```python
from build123d import *

# Parameters (mm, degrees)
F0_W     = 15
F0_H     = 25
F0_R     = 2.25
F1_DEPTH = 2.5
F2_W     = 15
F2_H     = 30
F2_R     = 2.25
F3_DEPTH = 5
F4_W     = 15
F4_H     = 30
F4_R     = 2.5
F5_DEPTH = 9


with BuildPart() as f1:
    # F0 (on Top) → F1 (new body)
    with BuildSketch(Plane.XY):
        with Locations((7.5, -12.5)):
            Rectangle(F0_W, F0_H)
        with Locations((7.5, -7.405)):
            Circle(F0_R, mode=Mode.SUBTRACT)
    extrude(amount=F1_DEPTH)

    # F2 (on face) → F3 (join)
    with BuildSketch(Plane.XY.offset(2.5)):
        with Locations((7.5, -15)):
            Rectangle(F2_W, F2_H)
        with Locations((7.5, -7.405)):
            Circle(F2_R, mode=Mode.SUBTRACT)
    extrude(amount=F3_DEPTH)

    # F4 (on face) → F5 (join)
    with BuildSketch(Plane(origin=(0, 0, 0), x_dir=(1, 0, 0), z_dir=(0, 0, -1))):
        with Locations((7.5, 15)):
            Rectangle(F4_W, F4_H)
        with Locations((7.5, 7.405)):
            Circle(F4_R, mode=Mode.SUBTRACT)
    extrude(amount=F5_DEPTH)


solid = f1.part
```
Design review of the part built by this model. Coordinates are the model's own, in mm. A direction names the side the tool comes from. Round coordinates to 2 decimals unless told otherwise and drop trailing zeros. Order: outer loops, then holes, each group sorted by start corner. A loop starts at its lowest first (then second) coordinate and runs counter-clockwise, first axis right, second up. Notation, with made-up numbers: (26, 28) - (77, 28) arc R10 cw to (77, 40) - close; hole circle Ø10 at (53, 54.5). An arc over 180 degrees is marked (long way). One line per question, with ' | ' between items.
Item 1: For P1, Ø0.8, axis at x = 4, z = 1, coming from the -Y side, flat-tipped, find the tip position at first contact; note if it passes through.
Checks:
P1: y = -25
Item 2: Take a section at B-B, the plane y = -9. Write out the cut boundary in (x, z), then the cut area to 3 significant figures.
Checks:
outline: (0, -9) - (5.57, -9) - (5.57, 0) - (5.91, 0) - (5.91, 7.5) - (0, 7.5) - close; (9.09, 0) - (9.43, 0) - (9.43, -9) - (15, -9) - (15, 7.5) - (9.09, 7.5) - close | area: 189 mm²
Item 3: Wall thickness on line 1 (Y direction, x = 7.5, z = 4) (3 decimals); line 2 (Y direction, x = 7.5, z = 2) (3 decimals); line 3 (Z direction, x = 11.75, y = -26.5): over which ranges is each line inside the solid? List them lowest first. Write a range as [from, to].
Checks:
line 1: [-30, -9.655], [-5.155, 0] | line 2: [-25, -9.655], [-5.155, 0] | line 3: [-9, 0], [2.5, 7.5]
Item 4: Machinability: for faces 4 (the face through (7, -30, -4)), 5 (the face through (7, -25, 1)), 6 (the face through (8.844, -9.513, -4.437)), which of the approach directions +Z, -Z, +X, -X, +Y, -Y give a long, thin tool a straight path to every point of the face, cutting with its end or side? Answer none if there is none.
Checks:
face 4: +Z, -Z, +X, -X, -Y | face 5: +X, -X, -Y | face 6: -Z
Item 5: Draft analysis for pull direction Z (two halves, no side actions). For faces 1 (the face through (0, -15, -1)), 2 (the face through (7, -15, 7.5)), 3 (the face through (7, -28, 0)), state which applies: +Z half, -Z half, draft (parallel to the pull), parting line (faces both ways), or undercut.
Checks:
face 1: draft | face 2: +Z half | face 3: undercut
Item 6: Take a section at A-A, the plane x = 7.5. Write out the cut boundary in (y, z) (3 decimals).
Checks:
outline: (-30, -9) - (-9.905, -9) - (-9.905, 0) - (-9.655, 0) - (-9.655, 7.5) - (-30, 7.5) - (-30, 2.5) - (-25, 2.5) - (-25, 0) - (-30, 0) - close; (-5.155, 0) - (-4.905, 0) - (-4.905, -9) - (0, -9) - (0, 7.5) - (-5.155, 7.5) - close
Item 7: Take a section at C-C, the plane z = -4.25. Write out the cut boundary in (x, y) (3 decimals).
Checks:
outline: (0, -30) - (15, -30) - (15, 0) - (0, 0) - close; hole circle Ø5 at (7.5, -7.405)
Item 8: Take a section at D-D, the plane x = 2.25. Write out the cut boundary in (y, z).
Checks:
outline: (-30, -9) - (0, -9) - (0, 7.5) - (-30, 7.5) - (-30, 2.5) - (-25, 2.5) - (-25, 0) - (-30, 0) - close
